from build123d import *

# Parameters (mm, degrees)
SKETCH_3_R          = 1.75
CUT_EXTRUDE_2_DEPTH = 211.5
SKETCH_4_R          = 5
CUT_EXTRUDE_3_DEPTH = 0.1


with BuildPart() as part:
    # Эскиз2 → Повернуть1 (revolve)
    with BuildSketch(Plane(origin=(0, 0, 0), x_dir=(1, 0, 0), z_dir=(0, 1, 0))):
        with BuildLine():
            Line((-135, 0), (-132, 0))
            ThreePointArc((-132, 0), (-93.338095117, 93.338095117), (0, 132))
            Line((0, 132), (0, 135))
            ThreePointArc((0, 135), (-95.45941546, 95.45941546), (-135, 0))
        make_face()
    revolve(axis=Axis((0, 0, -135), (0, 0, 1)))

    # Эскиз3 → Вырез-Вытянуть2 (cut, symmetric)
    with BuildSketch(Plane(origin=(0, 0, 0), x_dir=(0, -1, 0), z_dir=(1, 0, 0))):
        with Locations((9.192388155, 9.192388155)):
            Circle(SKETCH_3_R)
        with Locations((-9.192388155, 9.192388155)):
            Circle(SKETCH_3_R)
    extrude(amount=CUT_EXTRUDE_2_DEPTH, both=True, mode=Mode.SUBTRACT)

    # Эскиз4 → Вырез-Вытянуть3 (cut)
    with BuildSketch(Plane(origin=(135, 0, 0), x_dir=(0, 0, -1), z_dir=(1, 0, 0))):
        Circle(SKETCH_4_R)
    cut_extrude_3 = extrude(amount=-CUT_EXTRUDE_3_DEPTH, mode=Mode.SUBTRACT)

    # Зеркальное отражение1: Вырез-Вытянуть3 across plane
    add(cut_extrude_3.mirror(Plane(origin=(0, 0, 0), x_dir=(0, 0, 1), z_dir=(1, 0, 0))), mode=Mode.SUBTRACT)


solid = part.part
The listing builds one solid part. Answer for the finished solid, in the listing's coordinates (mm). Coordinates: 2 decimals unless noted, no trailing zeros. Loops run counter-clockwise (first coordinate to the right, second up) from the corner with the lowest first, then second, coordinate; pieces in that order, holes last.
1) Find section D-D on y = 44. Write down the section's boundary in (x, z).
2) Find the intervals of material crossed by L1, parallel to Y at x = 93, z = -9.5; L2, parallel to Y at x = 37, z = -104; L3, parallel to X at y = -63.5, z = -42.5, in increasing order.
3) Find section B-B on z = -49. Write down the section's boundary in (x, y), then the cut area to 3 significant figures.
4) Flat-ended cylindrical pins translate along their axes: pin 1 Ø3 at (y, z) = (-9.19, -9.19) entering from +X; pin 2 Ø6 at (y, z) = (-3, -70) entering from -X; pin 3 Ø5 at (x, z) = (52, -28.5) entering from +Y; pin 4 Ø4.5 at (y, z) = (9.19, -9.19) entering from -X. Find the tip coordinate at first contact, or state that the pin passes through.
5) Find section C-C on x = 11.5. Write down the section's boundary in (y, z).
Values:
1. outline: (-127.63, 0) arc R127.63 ccw to (127.63, 0) - (124.45, 0) arc R124.45 cw to (-124.45, 0) - close
2. L1: y = -97.39 to -93.19, 93.19 to 97.39
2. L2: y = -77.72 to -72.38, 72.38 to 77.72
2. L3: x = -111.29 to -107.64, 107.64 to 111.29
3. outline: circle Ø251.59 at (0, 0); hole circle Ø245.14 at (0, 0)
3. area: 2,520 mm2
4. pin 1: passes through
4. pin 2: stops at x = -117.16
4. pin 3: stops at y = 122.47
4. pin 4: stops at x = -134.57
5. outline: (-134.51, 0) arc R134.51 ccw to (134.51, 0) - (131.5, 0) arc R131.5 cw to (-131.5, 0) - close
